```python
from build123d import *

# Parameters (mm, degrees)
SKETCH1_W           = 12
SKETCH1_H           = 12
SKETCH1_R           = 2.475
BOSS_EXTRUDE1_DEPTH = 12
LPATTERN1_COUNT     = 5
LPATTERN1_PITCH     = 12
LPATTERN1_COL_COUNT = 2
LPATTERN1_COL_PITCH = 12
SKETCH2_R           = 3.05
SKETCH2_R_2         = 3.1
SKETCH2_R_3         = 3.15
SKETCH2_R_4         = 3.2
SKETCH2_R_5         = 3.25
SKETCH2_R_6         = 3.3
CUT_EXTRUDE1_DEPTH  = 5.75


with BuildPart() as part:
    # Sketch1 → Boss-Extrude1 (new body)
    with BuildSketch(Plane(origin=(0, 0, 0), x_dir=(1, 0, 0), z_dir=(0, 1, 0))):
        with Locations((6, 6)):
            Rectangle(SKETCH1_W, SKETCH1_H)
        with Locations(Location((6, 6, 0), (0, 0, 270))):
            Circle(SKETCH1_R, mode=Mode.SUBTRACT)
    boss_extrude1 = extrude(amount=BOSS_EXTRUDE1_DEPTH)

    # LPattern1: Boss-Extrude1 ×5
    with Locations(*[(-i * LPATTERN1_PITCH, 0, 0) for i in range(1, LPATTERN1_COUNT)]):
        add(boss_extrude1)


with BuildPart() as lpattern1_col_1:
    # LPattern1 col: Boss-Extrude1 ×2
    with Locations(*[(i * LPATTERN1_COL_PITCH, 0, 0) for i in range(1, LPATTERN1_COL_COUNT)]):
        add(boss_extrude1)


with BuildPart() as part_1:
    add(part.part)

    # LPattern1 col united with what the copie: union LPattern1 col_1
    add(lpattern1_col_1.part)

    # Sketch2 → Cut-Extrude1 (cut)
    with BuildSketch(Plane(origin=(0, 12, 0), x_dir=(1, 0, 0), z_dir=(0, 1, 0))):
        with Locations(Location((-42, 6, 0), (0, 0, 270))):
            Circle(SKETCH2_R)
        with Locations(Location((-30, 6, 0), (0, 0, 270))):
            Circle(SKETCH2_R_2)
        with Locations(Location((-18, 6, 0), (0, 0, 270))):
            Circle(SKETCH2_R_3)
        with Locations(Location((-6, 6, 0), (0, 0, 270))):
            Circle(SKETCH2_R_4)
        with Locations(Location((6, 6, 0), (0, 0, 270))):
            Circle(SKETCH2_R_5)
        with Locations(Location((18, 6, 0), (0, 0, 270))):
            Circle(SKETCH2_R_6)
    extrude(amount=-CUT_EXTRUDE1_DEPTH, mode=Mode.SUBTRACT)


solid = part_1.part
```
Source: CAD feature listing. Evaluate the final solid. Frame: model axes, mm. A direction names the side the tool comes from. Give positions to 0.01 mm unless a question says otherwise; leave off trailing zeros. Loops run counter-clockwise (first coordinate to the right, second up) from the corner with the lowest first, then second, coordinate; pieces in that order, holes last. Notation, with made-up numbers: (14.25, 75) - (38.25, 75) arc R11 cw to (38.25, 88) - close; hole circle Ø7 at (66.25, 30). An arc over 180 degrees is marked (long way). Use CSV: the item, a comma, the result in double quotes. Start each with the question number.
1. Ray query, L1, parallel to Z at x = -41.5, y = 7; L2, parallel to Z at x = -43, y = 10.5; L3, parallel to Y at x = -30.5, z = -8.5. Return the intervals inside material, ascending.
2. Pin query (flat end, axial travel): pin 1 (5 mm diameter, centred on x = 7.5, z = -5.5, fed in from +Y); pin 2 (2 mm diameter, centred on x = 19.5, z = -5.5, fed in from +Y). Return the tip coordinate at first contact, or that it passes through.
3. Section C-C (x = -30). Output: boundary loops of the cut face in (y, z) (3 decimals), then the cut area to 3 significant figures.
4. Draft query along Z for faces 3 (the flat face through (24, 6, -6)), 4 (the flat face through (-13, 6, 0)), 5 (the cylindrical face through (-44.977, 9.165, -6.661)). Return one class per face: +Z half, -Z half, draft (parallel to the pull), parting line (faces both ways), or undercut.
5. Section D-D (y = 4.5). Output: boundary loops of the cut face in (x, z) (3 decimals), then the cut area to 3 significant figures.
6. Section B-B (y = 10). Output: boundary loops of the cut face in (x, z), then the cut area to 3 significant figures.
7. Section A-A (x = -42). Output: boundary loops of the cut face in (y, z) (3 decimals), then the cut area to 3 significant figures.
8. Reachability of faces 1 (the cylindrical face through (5.052, 3.081, -3.714)), 2 (the flat face through (-8, 6.25, -4)) from +Z, -Z, +X, -X, +Y, -Y: full face, straight path, thin tool, end or side. Return the list, or none.
Response:
1,L1,"-12 to -9.01, -2.99 to 0"
1,L2,"-12 to -8.88, -3.12 to 0"
1,L3,"0 to 6.25"
2,pin 1,"y = 12"
2,pin 2,"y = 6.25"
3,outline,"(0, -12) - (12, -12) - (12, -9.1) - (6.25, -9.1) - (6.25, -8.475) - (0, -8.475) - close; (0, -3.525) - (6.25, -3.525) - (6.25, -2.9) - (12, -2.9) - (12, 0) - (0, 0) - close"
3,area,"77.4 mm²"
4,face 3,"draft"
4,face 4,"+Z half"
4,face 5,"undercut"
5,outline,"(-48, -12) - (24, -12) - (24, 0) - (-48, 0) - close; hole circle Ø4.95 at (-42, -6); hole circle Ø4.95 at (-30, -6); hole circle Ø4.95 at (-18, -6); hole circle Ø4.95 at (-6, -6); hole circle Ø4.95 at (6, -6); hole circle Ø4.95 at (18, -6)"
5,area,"749 mm²"
6,outline,"(-48, -12) - (24, -12) - (24, 0) - (-48, 0) - close; hole circle Ø6.1 at (-42, -6); hole circle Ø6.2 at (-30, -6); hole circle Ø6.3 at (-18, -6); hole circle Ø6.4 at (-6, -6); hole circle Ø6.5 at (6, -6); hole circle Ø6.6 at (18, -6)"
6,area,"674 mm²"
7,outline,"(0, -12) - (12, -12) - (12, -9.05) - (6.25, -9.05) - (6.25, -8.475) - (0, -8.475) - close; (0, -3.525) - (6.25, -3.525) - (6.25, -2.95) - (12, -2.95) - (12, 0) - (0, 0) - close"
7,area,"78.0 mm²"
8,face 1,"+Y, -Y"
8,face 2,"+Y"
